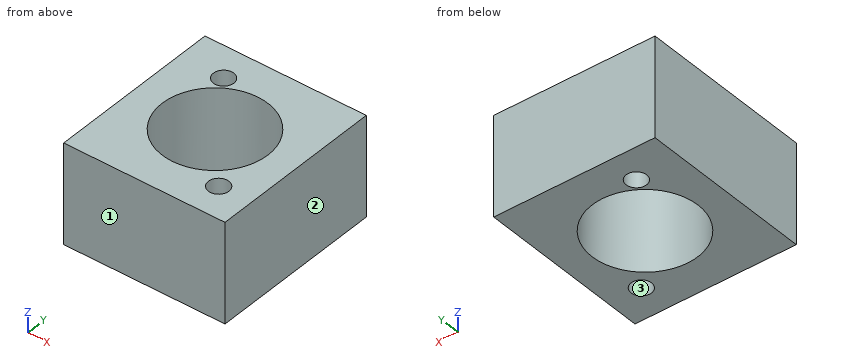
```python
from build123d import *

# Parameters (mm, degrees)
F0_W     = 25.019
F0_H     = 27.178
F0_W_2   = 19.939
F0_H_2   = 22.098
F0_R     = 1.5875
F0_R_2   = 8.1915
F1_DEPTH = 15.494


with BuildPart() as f1:
    # F0 (on Top) → F1 (new body)
    with BuildSketch(Plane.XY):
        Rectangle(F0_W, F0_H)
        Rectangle(F0_W_2, F0_H_2, mode=Mode.SUBTRACT)
        Rectangle(F0_W_2, F0_H_2)
        with Locations((7.4295, -8.509)):
            Circle(F0_R, mode=Mode.SUBTRACT)
        with Locations((-5.5245, 8.509)):
            Circle(F0_R, mode=Mode.SUBTRACT)
        Circle(F0_R_2, mode=Mode.SUBTRACT)
    extrude(amount=F1_DEPTH)


solid = f1.part
```
The listing builds one solid part. Answer for the finished solid, in the listing's coordinates (mm). Face numbers are marked on the shaded views. Coordinates: 2 decimals unless noted, no trailing zeros. Write each loop counter-clockwise with the first axis right and the second up, starting at its lowest first coordinate (ties: lowest second). Pieces come first, ordered by that corner, then holes. Notation, with made-up numbers: (11, 88) - (34, 88) arc R28 ccw to (34, 127) - close; hole circle Ø2 at (-14, 7). An arc over 180 degrees is marked (long way). One line per item, written item: value.
1) Find section C-C (z = 13.25). Give the vertices of the cut face in (x, y) (1 decimal), and give its area (3 significant figures).
Geometry check:
outline: (-12.5, -13.6) - (12.5, -13.6) - (12.5, 13.6) - (-12.5, 13.6) - close; hole circle Ø16.4 at (0, 0); hole circle Ø3.2 at (-5.5, 8.5); hole circle Ø3.2 at (7.4, -8.5)
area: 453 mm2
2) This flat-tipped pin is pushed along its axis until it touches: pin 1 Ø8 at (x, y) = (0.5, -7) entering from -Z. Where does it stop, or does it pass through?
Geometry check:
pin 1: stops at z = 0
3) For a pull along X with two mould halves and no side action, classify the marked faces 1, 2 and 3 as pulls with the +X half, pulls with the -X half, needs draft (parallel to the pull), parting line crosses it, or undercut.
Geometry check:
face 1: needs draft
face 2: pulls with the +X half
face 3: undercut
4) Find section A-A (y = 0). Give the vertices of the cut face in (x, z), and give its area (3 significant figures).
Geometry check:
outline: (-12.51, 0) - (-8.19, 0) - (-8.19, 15.49) - (-12.51, 15.49) - close; (8.19, 0) - (12.51, 0) - (12.51, 15.49) - (8.19, 15.49) - close
area: 134 mm2
5) Consider line 1 along Y through (x, z) = (0, 12.25); line 2 along X through (y, z) = (-0.25, 9); line 3 along Y through (x, z) = (-6.5, 10.25). Determine where each line is inside the solid, lowest interval first. Write a range as from..to.
Geometry check:
line 1: y = -13.59..-8.19, 8.19..13.59
line 2: x = -12.51..-8.19, 8.19..12.51
line 3: y = -13.59..-4.99, 4.99..7.26, 9.76..13.59
6) Find section B-B (x = 0). Give the vertices of the cut face in (y, z), and give its area (3 significant figures).
Geometry check:
outline: (-13.59, 0) - (-8.19, 0) - (-8.19, 15.49) - (-13.59, 15.49) - close; (8.19, 0) - (13.59, 0) - (13.59, 15.49) - (8.19, 15.49) - close
area: 167 mm2
